Design review of the part built by this model. Coordinates are the model's own, in mm. A direction names the side the tool comes from. Coordinates: 2 decimals unless noted, no trailing zeros. Order: outer loops, then holes, each group sorted by start corner. A loop starts at its lowest first (then second) coordinate and runs counter-clockwise, first axis right, second up.
Autodesk Inventor part; units mm, degrees
ref_plane "YZ Plane" through (0, 0, 0) normal (1, 0, 0) x (0, 1, 0)
ref_plane "XZ Plane" through (0, 0, 0) normal (0, 1, 0) x (-1, 0, 0)
ref_plane "XY Plane" through (0, 0, 0) normal (0, 0, 1) x (1, 0, 0)
sketch "Sketch1" plane through (0, 0, 0) normal (0, 0, 1) x (1, 0, 0)
  circle A0 centre (0, 0) radius 2.5
  dimension "d0" = 5
extrude "Extrusion1" add sketch "Sketch1" against normal blind 40
sketch "Sketch2" plane through (0, 0, 0) normal (0, 0, 1) x (1, 0, 0)
  circle A0 centre (0, 0) radius 4.3
  dimension "d3" = 8.6
extrude "Extrusion2" add sketch "Sketch2" along normal blind 4
fillet "Fillet1" radius 2 1 edges at (-4.3, 0, 4)
sketch "Sketch3" plane through (0, 0, 4) normal (0, 0, 1) x (1, 0, 0)
  line L0 (0, -2.162) -> (-1.8723, -1.081)
  line L1 (-1.8723, -1.081) -> (-1.8723, 1.081)
  line L2 (-1.8723, 1.081) -> (0, 2.162)
  line L3 (0, 2.162) -> (1.8723, 1.081)
  line L4 (1.8723, 1.081) -> (1.8723, -1.081)
  line L5 (1.8723, -1.081) -> (0, -2.162)
  point P0 (0, 0)
  point P1 (0, 0)
extrude "Extrusion3" cut sketch "Sketch3" against normal blind 0.5
chamfer "Chamfer1" distance 0.5 angle 45 1 edges at (-2.5, 0, -40)
properties part number "bolt m5"
1. Add section A-A (y = 0). Give the boundary of the cut face in (x, z), and give its area (3 significant figures).
2. Add section B-B (z = -37). Give the boundary of the cut face in (x, y), and give its area (3 significant figures).
3. For faces 1 (the flat face through (0.949, -1.614, 3.754)), 2 (the flat face through (0, 0, -40)), list the 3-axis set-ups (+Z, -Z, +X, -X, +Y, -Y) from which the entire face can be reached by the end or side of a thin tool; tool diameter is ignored.
4. Mouldability with a two-part tool opening along Y and no side actions: class faces 3 (the cylindrical face through (-0.54, -2.44, -19.47)), 4 (the flat face through (-0.92, -1.63, 3.75)), 5 (the flat face through (2, -2, 0)) as pulls with the +Y half, pulls with the -Y half, needs draft (parallel to the pull), parting line crosses it, or undercut.
5. To check wall thickness, follow line 1 (Z direction, x = 0, y = 1); line 2 (X direction, y = 1.5, z = -16.5); line 3 (X direction, y = 2.25, z = -5.5). State the ranges of each line that lie inside material, in increasing order.
6. Insertion check: pin 1 (4 mm diameter, centred on x = -3, y = -0.5, fed in from +Z); pin 2 (1.9 mm diameter, centred on x = 0, y = -0.5, fed in from +Z); pin 3 (1.5 mm diameter, centred on y = 0, z = -9, fed in from +X); pin 4 (5 mm diameter, centred on x = -3, z = -20, fed in from -Y). Each pin has a flat end and moves straight along its axis. Give the tip position at first contact, or say it passes through.
Solution:
1. outline: (-4.3, 0) - (-2.5, 0) - (-2.5, -39.5) - (-2, -40) - (2, -40) - (2.5, -39.5) - (2.5, 0) - (4.3, 0) - (4.3, 2) arc R2 ccw to (2.3, 4) - (1.87, 4) - (1.87, 3.5) - (-1.87, 3.5) - (-1.87, 4) - (-2.3, 4) arc R2 ccw to (-4.3, 2) - close
1. area: 231 mm2
2. outline: circle Ø5 at (0, 0)
2. area: 19.6 mm2
3. face 1: +Z
3. face 2: -Z, +X, -X, +Y, -Y
4. face 3: parting line crosses it
4. face 4: undercut
4. face 5: needs draft
5. line 1: z = -40 to 3.5
5. line 2: x = -2 to 2
5. line 3: x = -1.09 to 1.09
6. pin 1: stops at z = 4
6. pin 2: stops at z = 3.5
6. pin 3: stops at x = 2.5
6. pin 4: stops at y = -2.45
